```python
from build123d import *

# Parameters (mm, degrees)
F0_R     = 23.495
F1_DEPTH = 6.35
F2_R     = 3.81
F3_DEPTH = 28.575
F4_SIZE  = 0.508


with BuildPart() as f1:
    # F0 (on Top) → F1 (new body)
    with BuildSketch(Plane.XY):
        with BuildLine():
            ThreePointArc((-141.924887, 7.453309), (-135.89, 0), (-141.924887, -7.453309))
            Line((-141.924887, -7.453309), (-151.954259, -9.586279))
            ThreePointArc((-151.954259, -9.586279), (-155.087703, -13.654877), (-151.573483, -17.399504))
            Line((-151.573483, -17.399504), (-77.281462, -25.767059))
            ThreePointArc((-77.281462, -25.767059), (-42.510822, -42.510822), (-25.767059, -77.281462))
            Line((-25.767059, -77.281462), (-17.399504, -151.573483))
            ThreePointArc((-17.399504, -151.573483), (-13.654877, -155.087703), (-9.586279, -151.954259))
            Line((-9.586279, -151.954259), (-7.453309, -141.924887))
            ThreePointArc((-7.453309, -141.924887), (0, -135.89), (7.453309, -141.924887))
            Line((7.453309, -141.924887), (9.586279, -151.954259))
            ThreePointArc((9.586279, -151.954259), (13.654877, -155.087703), (17.399504, -151.573483))
            Line((17.399504, -151.573483), (25.767059, -77.281462))
            ThreePointArc((25.767059, -77.281462), (42.510822, -42.510822), (77.281462, -25.767059))
            Line((77.281462, -25.767059), (151.573483, -17.399504))
            ThreePointArc((151.573483, -17.399504), (155.087703, -13.654877), (151.954259, -9.586279))
            Line((151.954259, -9.586279), (141.924887, -7.453309))
            ThreePointArc((141.924887, -7.453309), (135.89, 0), (141.924887, 7.453309))
            Line((141.924887, 7.453309), (151.954259, 9.586279))
            ThreePointArc((151.954259, 9.586279), (155.087703, 13.654877), (151.573483, 17.399504))
            Line((151.573483, 17.399504), (77.281462, 25.767059))
            ThreePointArc((77.281462, 25.767059), (42.510822, 42.510822), (25.767059, 77.281462))
            Line((25.767059, 77.281462), (17.399504, 151.573483))
            ThreePointArc((17.399504, 151.573483), (13.654877, 155.087703), (9.586279, 151.954259))
            Line((9.586279, 151.954259), (7.453309, 141.924887))
            ThreePointArc((7.453309, 141.924887), (0, 135.89), (-7.453309, 141.924887))
            Line((-7.453309, 141.924887), (-9.586279, 151.954259))
            ThreePointArc((-9.586279, 151.954259), (-13.654877, 155.087703), (-17.399504, 151.573483))
            Line((-17.399504, 151.573483), (-25.767059, 77.281462))
            ThreePointArc((-25.767059, 77.281462), (-42.510822, 42.510822), (-77.281462, 25.767059))
            Line((-77.281462, 25.767059), (-151.573483, 17.399504))
            ThreePointArc((-151.573483, 17.399504), (-155.087703, 13.654877), (-151.954259, 9.586279))
            Line((-151.954259, 9.586279), (-141.924887, 7.453309))
        make_face()
        Circle(F0_R, mode=Mode.SUBTRACT)
    extrude(amount=F1_DEPTH)

    # F2 (on face) → F3 (join)
    with BuildSketch(Plane.XY.offset(6.35)):
        with Locations((-44.45, 0)):
            Circle(F2_R)
        with Locations((44.45, 0)):
            Circle(F2_R)
    extrude(amount=F3_DEPTH)

    # F4
    f4_edges = [f1.edges().sort_by_distance(p)[0] for p in [
        (-48.26, 0, 34.925),
        (40.64, 0, 34.925),
    ]]
    chamfer(f4_edges, length=F4_SIZE)


solid = f1.part
```
Here's how the part is built. I have some questions about the finished solid (model axes, mm). A direction names the side the tool comes from. Give positions to 0.01 mm unless a question says otherwise; leave off trailing zeros. Loops run counter-clockwise (first coordinate to the right, second up) from the corner with the lowest first, then second, coordinate; pieces in that order, holes last. Notation, with made-up numbers: M -32.75,-27.75 L 9.25,-27.75 A14 cw 9.25,-6.75 Z; hole C -24.5,36 d4. An arc over 180 degrees is marked long. Use one line per item in the form item = value. Start each with the question number.
Q1. If we section it at A-A (z = 29): Write out the boundary of the cut face in (x, y), then the cut area to 3 significant figures.
Q2. If we section it at C-C (y = -92.5): Write out the boundary of the cut face in (x, z), then the cut area to 3 significant figures.
Q3. Thinking about a two-plate mould opening in Y: for faces 3 (the cylindrical face through (40.644, 0.168, 20.187)), 4 (the cylindrical face through (-5.093, -22.936, 3.131)), 5 (the flat face through (-21.525, 114.948, 3.131)), 6 (the flat face through (-114.948, -21.525, 3.131)), which applies, +Y half, -Y half, draft (parallel to the pull), parting line (faces both ways), or undercut?
Q4. If we section it at B-B (x = -67.5): Write out the boundary of the cut face in (y, z), then the cut area to 3 significant figures.
Q5. Will these pins go through, and if not, where does the flat tip stop? pin 1 Ø4 at (y, z) = (-102, 5.5) entering from +X; pin 2 Ø5 at (x, z) = (-84, 8) entering from +Y; pin 3 Ø2 at (y, z) = (2, 3.5) entering from +X.
Q6. Which directions (+Z, -Z, +X, -X, +Y, -Y) give clear straight access to the entire face, cutting with the end or side of a thin tool? Please do faces 1 (the cylindrical face through (-48.256, 0.168, 20.187)), 2 (the flat face through (21.525, -114.948, 3.131)).
Q7. I need wall thicknesses on line 1 along Y through (x, z) = (0, 3.75) (3 decimals); line 2 along Z through (x, y) = (15.5, 86.5); line 3 along Y through (x, z) = (42.5, 25.5). Which ranges of each line are inside material? Lowest first, please.
Taken from the geometry:
q1.outline = C -44.45,0 d7.62; C 44.45,0 d7.62
q1.area = 91.2 mm^2
q2.outline = M -24.05,0 L 24.05,0 L 24.05,6.35 L -24.05,6.35 Z
q2.area = 305 mm^2
q3.face_3 = parting line
q3.face_4 = undercut
q3.face_5 = +Y half
q3.face_6 = -Y half
q4.outline = M -27.73,0 L 27.73,0 L 27.73,6.35 L -27.73,6.35 Z
q4.area = 352 mm^2
q5.pin_1 = 23.21
q5.pin_2 = 25.22
q5.pin_3 = 136.51
q6.face_1 = +Z
q6.face_2 = +Z, -Z, +X, -Y
q7.line_1 = -135.89 to -23.495, 23.495 to 135.89
q7.line_2 = 0 to 6.35
q7.line_3 = -3.27 to 3.27
